Check sheet for the drawn part. Datum: minimum x, y, z corner. Units: mm. A direction names the side the tool comes from. Coordinates: 2 decimals unless noted, no trailing zeros. Loops run counter-clockwise (first coordinate to the right, second up) from the corner with the lowest first, then second, coordinate; pieces in that order, holes last. Notation, with made-up numbers: M -36,-2 L 9,-2 A19 cw 9,10 Z; hole C 86.5,-22.5 d11. An arc over 180 degrees is marked long. Use CSV: the item, a comma, the result in double quotes. Start each with the question number.
(1) Set-up check for the marked faces 4 and 5: record each of +Z, -Z, +X, -X, +Y, -Y from which the full face is reachable in a straight line by a thin tool's end or side.
(2) Scan lines: line 1 (X direction, y = 19, z = 68); line 2 (Z direction, x = 55, y = 19.7); line 3 (X direction, y = 14.5, z = 16.5). Record each from-to range of solid material in increasing order.
(3) Draft check along X on the marked faces 1, 2 and 3. Enter one of: pulls with the +X half, pulls with the -X half, needs draft (parallel to the pull), parting line crosses it, or undercut.
(4) Section check B-B on y = 8.5. Record the cut outline in (x, z), and give its area (3 significant figures).
(5) Go/stop test with flat-tipped pins: pin 1 Ø8.5 at (x, z) = (55, 69) entering from +Y; pin 2 Ø3 at (x, y) = (59.5, 11) entering from +Z; pin 3 Ø2.5 at (x, z) = (55, 68) entering from +Y; pin 4 Ø2 at (x, y) = (32, 27.5) entering from -Z. Record where each tip stops, or that it passes through.
(6) Section check C-C on x = 37.5. Record the cut outline in (y, z).
(7) Section check D-D on y = 4. Record the cut outline in (x, z).
(8) Section check A-A on y = 17.5. Give the number of separate pieces and of enclosed holes in the cut face, and give its area (3 significant figures).
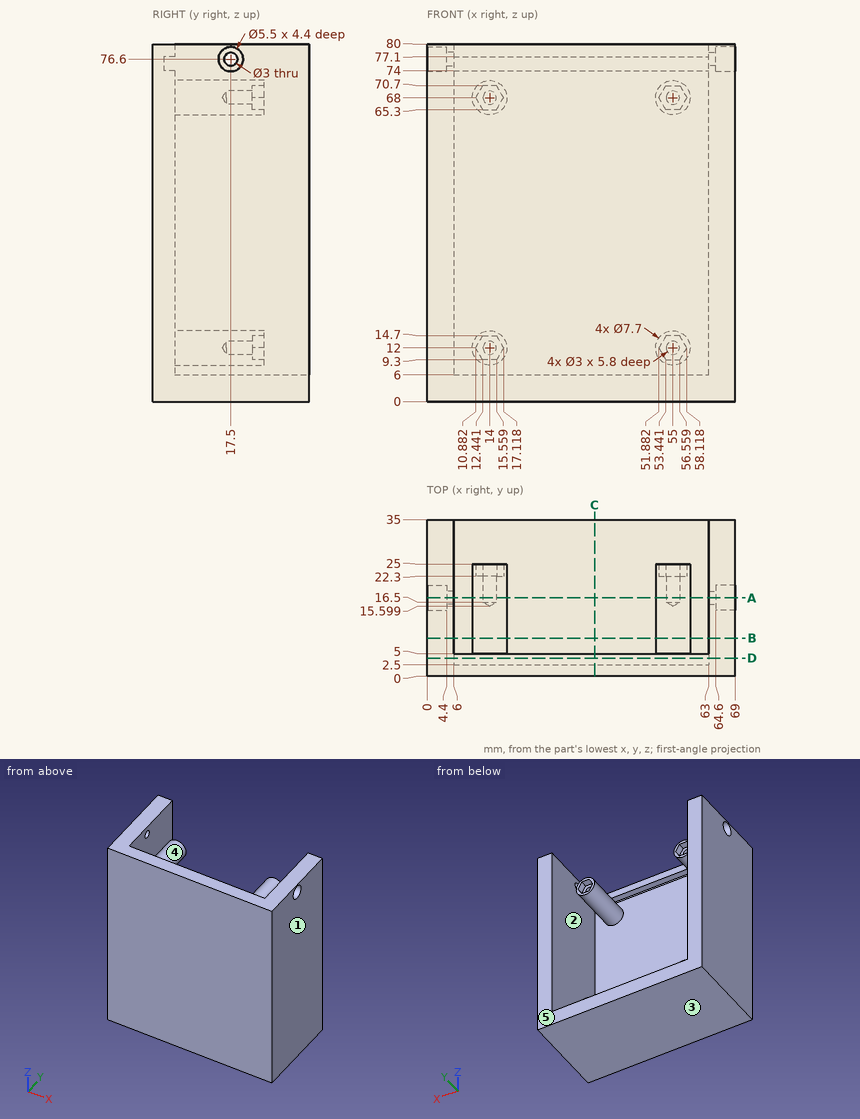
Outcome:
1,face 4,"+Y"
1,face 5,"+Z, -Z, +X, -X, +Y"
2,line 1,"x = 0 to 6, 10.15 to 12.5, 15.5 to 17.85, 51.15 to 53.5, 56.5 to 58.85, 63 to 69"
2,line 2,"z = 0 to 6, 8.15 to 10.5, 13.5 to 15.85, 64.15 to 66.5, 69.5 to 71.85"
2,line 3,"x = 0 to 6, 63 to 69"
3,face 1,"pulls with the +X half"
3,face 2,"undercut"
3,face 3,"needs draft"
4,outline,"M 0,0 L 69,0 L 69,80 L 63,80 L 63,6 L 6,6 L 6,80 L 0,80 Z; C 14,12 d7.7; C 14,68 d7.7; C 55,12 d7.7; C 55,68 d7.7"
4,area,"1,490 mm²"
5,pin 1,"stops at y = 25"
5,pin 2,"stops at z = 70.41"
5,pin 3,"stops at y = 16.35"
5,pin 4,"stops at z = 0"
6,outline,"M 0,0 L 35,0 L 35,6 L 5,6 L 5,74 L 2.5,74 L 2.5,77.1 L 5,77.1 L 5,80 L 0,80 Z"
7,outline,"M 0,0 L 69,0 L 69,80 L 0,80 Z; hole M 6,74 L 63,74 L 63,77.1 L 6,77.1 Z"
8,separate pieces,"7"
8,enclosed holes,"4"
8,area,"1,400 mm²"
